Job drawing, mm, ordinate dimensions from the low corner. One solid piece. A direction names the side the tool comes from. Give positions to 0.01 mm unless a question says otherwise; leave off trailing zeros. Write each loop counter-clockwise with the first axis right and the second up, starting at its lowest first coordinate (ties: lowest second). Pieces come first, ordered by that corner, then holes. Notation, with made-up numbers: (-34, -18.5) - (-21, -18.5) arc R27 cw to (-21, 13.5) - close; hole circle Ø10 at (-33.5, 55.5). An arc over 180 degrees is marked (long way). Answer as a JSON object with one key per item and string values.
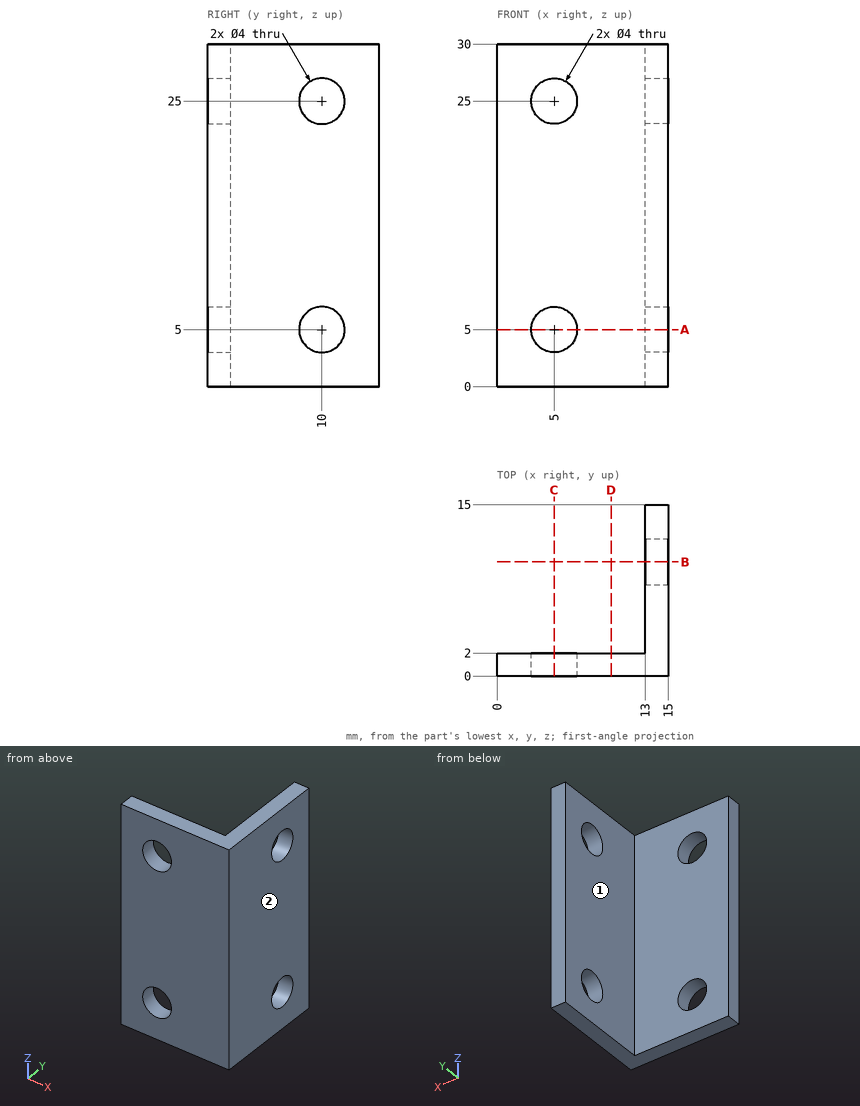
Item 1: Flat gauge pins, fed straight in: P1, Ø4.5, axis at y = 10, z = 25, coming from the -X side; P2, Ø3.5, axis at x = 5, z = 25, coming from the +Y side. Where does each tip first touch, or does it go through?
Entries:
{"P1": "x = 13", "P2": "through"}
Item 2: Cut at D-D (x = 10). Give the cut face in (y, z).
Entries:
{"outline": "(0, 0) - (2, 0) - (2, 30) - (0, 30) - close"}
Item 3: Probe line 1 (X direction, y = 1.15, z = 5); line 2 (Z direction, x = 5, y = 1.05); line 3 (Z direction, x = 4.5, y = 1). List the from-to ranges inside material, lowest first. Write a range as from..to.
Entries:
{"line 1": "0..3, 7..15", "line 2": "0..3, 7..23, 27..30", "line 3": "0..3.06, 6.94..23.06, 26.94..30"}
Item 4: Cut at B-B (y = 10). Give the cut face in (x, z).
Entries:
{"outline": "(13, 0) - (15, 0) - (15, 3) - (13, 3) - close; (13, 7) - (15, 7) - (15, 23) - (13, 23) - close; (13, 27) - (15, 27) - (15, 30) - (13, 30) - close"}
Item 5: Cut at C-C (x = 5). Give the cut face in (y, z), and give its area (3 significant figures).
Entries:
{"outline": "(0, 0) - (2, 0) - (2, 3) - (0, 3) - close; (0, 7) - (2, 7) - (2, 23) - (0, 23) - close; (0, 27) - (2, 27) - (2, 30) - (0, 30) - close", "area": "44.0 mm2"}
Item 6: Which spindle directions (+Z, -Z, +X, -X, +Y, -Y) get a long thin tool onto all of the face, cutting with end or side? Do the marked faces 1 and 2. Say none if no direction does.
Entries:
{"face 1": "+Z, -Z, -X, +Y", "face 2": "+Z, -Z, +X, +Y, -Y"}
Item 7: Cut at A-A (z = 5). Give the cut face in (x, y).
Entries:
{"outline": "(0, 0) - (3, 0) - (3, 2) - (0, 2) - close; (7, 0) - (15, 0) - (15, 8) - (13, 8) - (13, 2) - (7, 2) - close; (13, 12) - (15, 12) - (15, 15) - (13, 15) - close"}
